Geometry: final body of the model. Coordinates: model frame, mm. Face numbers are marked on the shaded views. A direction names the side the tool comes from. Give positions to 0.01 mm unless a question says otherwise; leave off trailing zeros. Write each loop counter-clockwise with the first axis right and the second up, starting at its lowest first coordinate (ties: lowest second). Pieces come first, ordered by that corner, then holes. Notation, with made-up numbers: (7.5, 54.5) - (20.5, 54.5) arc R18 ccw to (20.5, 84.5) - close; hole circle Ø8 at (18.5, 87.25). An arc over 180 degrees is marked (long way). Use CSV: the item, a comma, the result in double quotes. Start each with the question number.
(1) Line query: probe 1 along X at (y, z) = (-64.25, 45); probe 2 along Z at (x, y) = (32, -62.5); probe 3 along Y at (x, z) = (0, -5.5). Output: solid intervals per line, ascending. Write a range as [from, to].
(2) First-contact query: pin 1 Ø15 at (x, z) = (-1.5, 26.5) entering from +Y; pin 2 Ø6 at (y, z) = (-42, 14) entering from -X; pin 3 Ø3 at (x, z) = (32, 10) entering from +Y; pin 4 Ø23 at (y, z) = (-41.5, 15) entering from +X. Flat tips, straight axial feed; report the tip coordinate or a pass-through.
(3) Draft query along X for the marked faces 4, 5 and 6. Return one class per face: released by +X, released by -X, zero draft, split by the parting line, or undercut.
(4) Section A-A on x = 0. Output: boundary loops of the cut face in (y, z), and give its area (3 significant figures).
(5) Reachability of the marked faces 1, 2 and 3 from +Z, -Z, +X, -X, +Y, -Y: full face, straight path, thin tool, end or side. Return the list, or none.
(6) Section D-D on y = -43. Output: boundary loops of the cut face in (x, z).
(7) Section C-C on y = -7.5. Output: boundary loops of the cut face in (x, z), and give its area (3 significant figures).
(8) Section B-B on y = 3. Output: boundary loops of the cut face in (x, z), and give its area (3 significant figures).
from build123d import *

# Parameters (mm, degrees)
SKETCH1_R           = 1.65
SKETCH1_R_2         = 11
BOSS_EXTRUDE1_DEPTH = 10
SKETCH2_W           = 80
SKETCH2_H           = 10
BOSS_EXTRUDE2_DEPTH = 10
SKETCH3_W           = 80
SKETCH3_H           = 10
BOSS_EXTRUDE3_DEPTH = 55
SKETCH4_W           = 8
SKETCH4_H           = 35
BOSS_EXTRUDE4_DEPTH = 30
CUT_EXTRUDE1_DEPTH  = 157
CUT_EXTRUDE2_DEPTH  = 157
FILLET1_R           = 5


with BuildPart() as part:
    # Sketch1 → Boss-Extrude1 (new body)
    with BuildSketch(Plane.XY):
        with BuildLine():
            ThreePointArc((21.680728295, 6.016312875), (6.9e-07, 22.5), (-21.680727926, 6.016314205))
            Line((-21.680727926, 6.016314205), (-40, -60))
            Line((-40, -60), (40, -60))
            Line((40, -60), (21.680728295, 6.016312875))
        make_face()
        with Locations((0, 15)):
            Circle(SKETCH1_R, mode=Mode.SUBTRACT)
        with Locations((-12.990381057, -7.5)):
            Circle(SKETCH1_R, mode=Mode.SUBTRACT)
        with Locations((12.990381057, -7.5)):
            Circle(SKETCH1_R, mode=Mode.SUBTRACT)
        Circle(SKETCH1_R_2, mode=Mode.SUBTRACT)
    extrude(amount=-BOSS_EXTRUDE1_DEPTH)

    # Sketch2 → Boss-Extrude2 (add)
    with BuildSketch(Plane(origin=(0, -60, 0), x_dir=(-1, 0, 0), z_dir=(0, -1, 0))):
        with Locations((0, 5)):
            Rectangle(SKETCH2_W, SKETCH2_H)
    extrude(amount=BOSS_EXTRUDE2_DEPTH)

    # Sketch3 → Boss-Extrude3 (add)
    with BuildSketch(Plane.XY):
        with Locations((0, -65)):
            Rectangle(SKETCH3_W, SKETCH3_H)
    extrude(amount=BOSS_EXTRUDE3_DEPTH)

    # Sketch4 → Boss-Extrude4 (add)
    with BuildSketch(Plane(origin=(0, -60, 0), x_dir=(1, 0, 0), z_dir=(0, 1, 0))):
        with Locations((-21, -17.5)):
            Rectangle(SKETCH4_W, SKETCH4_H)
        with Locations((21, -17.5)):
            Rectangle(SKETCH4_W, SKETCH4_H)
    extrude(amount=BOSS_EXTRUDE4_DEPTH)

    # Sketch5 → Cut-Extrude1 (cut)
    with BuildSketch(Plane.ZY.offset(25)):
        Polygon((0, -30), (35, -60), (35, -30), align=None)
    extrude(amount=-CUT_EXTRUDE1_DEPTH, mode=Mode.SUBTRACT)

    # Sketch6 → Cut-Extrude2 (cut)
    with BuildSketch(Plane(origin=(0, -60, 0), x_dir=(1, 0, 0), z_dir=(0, 1, 0))):
        with BuildLine():
            ThreePointArc((-33.75, -45), (-33.237436867, -46.237436867), (-32, -46.75))
            Line((-32, -46.75), (-32, -45))
            Line((-32, -45), (-33.75, -45))
        make_face()
        with BuildLine():
            Line((-32, -45), (-32, -46.75))
            ThreePointArc((-32, -46.75), (-30.762563133, -46.237436867), (-30.25, -45))
            ThreePointArc((-30.25, -45), (-32, -43.25), (-33.75, -45))
            Line((-33.75, -45), (-32, -45))
        make_face()
        with BuildLine():
            ThreePointArc((33.75, -45), (30.762563133, -43.762563133), (32, -46.75))
            Line((32, -46.75), (32, -45))
            Line((32, -45), (33.75, -45))
        make_face()
        with BuildLine():
            Line((32, -45), (32, -46.75))
            ThreePointArc((32, -46.75), (33.237436867, -46.237436867), (33.75, -45))
            Line((33.75, -45), (32, -45))
        make_face()
        with BuildLine():
            ThreePointArc((33.75, -10), (33.237436867, -8.762563133), (32, -8.25))
            Line((32, -8.25), (32, -10))
            Line((32, -10), (33.75, -10))
        make_face()
        with BuildLine():
            Line((32, -10), (32, -8.25))
            ThreePointArc((32, -8.25), (30.762563133, -11.237436867), (33.75, -10))
            Line((33.75, -10), (32, -10))
        make_face()
        with BuildLine():
            ThreePointArc((-30.25, -10), (-30.762563133, -8.762563133), (-32, -8.25))
            Line((-32, -8.25), (-32, -10))
            Line((-32, -10), (-33.75, -10))
            ThreePointArc((-33.75, -10), (-32, -11.75), (-30.25, -10))
        make_face()
        with BuildLine():
            Line((-32, -10), (-32, -8.25))
            ThreePointArc((-32, -8.25), (-33.237436867, -8.762563133), (-33.75, -10))
            Line((-33.75, -10), (-32, -10))
        make_face()
    extrude(amount=-CUT_EXTRUDE2_DEPTH, mode=Mode.SUBTRACT)

    # Fillet1
    fillet1_edges = [part.edges().sort_by_distance(p)[0] for p in [
        (32.5, -60, 0),
        (0, -60, 0),
        (-32.5, -60, 0),
        (-21, -60, 35),
        (-17, -60, 17.5),
        (-17, -45, 0),
        (-25, -60, 17.5),
        (-25, -45, 0),
        (-21, -30, 0),
        (17, -45, 0),
        (25, -45, 0),
        (21, -30, 0),
        (17, -60, 17.5),
        (25, -60, 17.5),
        (21, -60, 35),
    ]]
    fillet(fillet1_edges, radius=FILLET1_R)


solid = part.part
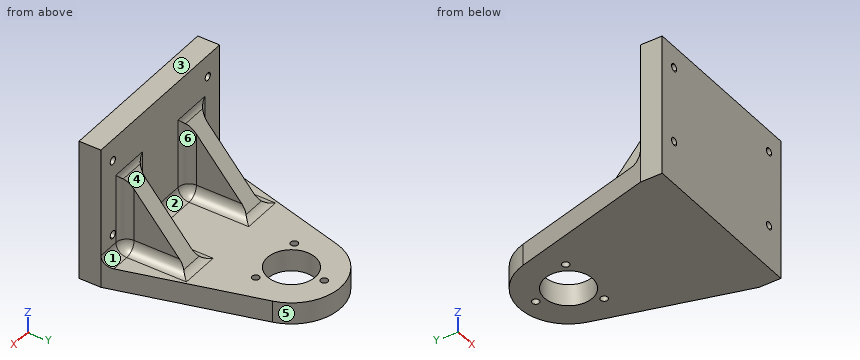
Check values:
1,probe 1,"x = [-40, -33.75], [-30.25, 30.25], [33.75, 40]"
1,probe 2,"z = [-10, 8.25], [11.75, 43.25], [46.75, 55]"
1,probe 3,"y = [-70, -11], [11, 13.35], [16.65, 22.5]"
2,pin 1,"stops at y = -60"
2,pin 2,"stops at x = -25"
2,pin 3,"passes through"
2,pin 4,"stops at x = 25.23"
3,face 4,"zero draft"
3,face 5,"split by the parting line"
3,face 6,"undercut"
4,outline,"(-70, -10) - (-11, -10) - (-11, 0) - (-55, 0) arc R5 cw to (-60, 5) - (-60, 55) - (-70, 55) - close; (11, -10) - (13.35, -10) - (13.35, 0) - (11, 0) - close; (16.65, -10) - (22.5, -10) - (22.5, 0) - (16.65, 0) - close"
4,area,"1,230 mm²"
5,face 1,"+Z, +X, +Y"
5,face 2,"+Z, +Y"
5,face 3,"+Z, +X, -X, +Y, -Y"
6,outline,"(-35.28, -10) - (35.28, -10) - (35.28, 0) - (30, 0) arc R5 cw to (25, 5) - (25, 15.17) - (17, 15.17) - (17, 5) arc R5 cw to (12, 0) - (-12, 0) arc R5 cw to (-17, 5) - (-17, 15.17) - (-25, 15.17) - (-25, 5) arc R5 cw to (-30, 0) - (-35.28, 0) - close"
7,outline,"(-25.43, -10) - (-14.64, -10) - (-14.64, 0) - (-25.43, 0) - close; (-11.34, -10) - (-8.05, -10) - (-8.05, 0) - (-11.34, 0) - close; (8.05, -10) - (11.34, -10) - (11.34, 0) - (8.05, 0) - close; (14.64, -10) - (25.43, -10) - (25.43, 0) - (14.64, 0) - close"
7,area,"282 mm²"
8,outline,"(-22.52, -10) - (-10.58, -10) - (-10.58, 0) - (-22.52, 0) - close; (10.58, -10) - (22.52, -10) - (22.52, 0) - (10.58, 0) - close"
8,area,"239 mm²"
